The listing builds one solid part. Answer for the finished solid, in the listing's coordinates (mm). A direction names the side the tool comes from. Coordinates: 2 decimals unless noted, no trailing zeros. Order: outer loops, then holes, each group sorted by start corner. A loop starts at its lowest first (then second) coordinate and runs counter-clockwise, first axis right, second up. Notation, with made-up numbers: (29, 26.5) -> (63, 26.5) arc R22 cw to (63, 33.5) -> close; hole circle Ø3 at (74, 74.5). An arc over 180 degrees is marked (long way). One line per question, with ' | ' between items.
from build123d import *

# Parameters (mm, degrees)
F1_DEPTH = 5
F3_DEPTH = 185


with BuildPart() as f1:
    # F0 (on Front) → F1 (new body)
    with BuildSketch(Plane.XZ):
        with BuildLine():
            ThreePointArc((185, 30), (179.1421356237, 44.1421356237), (165, 50))
            Line((165, 50), (-165, 50))
            ThreePointArc((-165, 50), (-179.1421356237, 44.1421356237), (-185, 30))
            Line((-185, 30), (-185, -50))
            Line((-185, -50), (185, -50))
            Line((185, -50), (185, 30))
        make_face()
    extrude(amount=F1_DEPTH)

    # F2 (on Right) → F3 (join, symmetric)
    with BuildSketch(Plane.YZ):
        with BuildLine():
            ThreePointArc((12.3411369137, -50.3849132597), (12.1417214903, -49.9034818398), (11.6602900704, -49.7040664163))
            Line((11.6602900704, -49.7040664163), (-16.9780162429, -49.7040664163))
            ThreePointArc((-16.9780162429, -49.7040664163), (-17.4594476628, -49.9034818398), (-17.6588630863, -50.3849132597))
            Line((-17.6588630863, -50.3849132597), (-17.6588630863, -52.7040664163))
            Line((-17.6588630863, -52.7040664163), (12.3411369137, -52.7040664163))
            Line((12.3411369137, -52.7040664163), (12.3411369137, -50.3849132597))
        make_face()
    extrude(amount=F3_DEPTH, both=True)


solid = f1.part
Item 1: Section B-B, the plane z = 22.5 is taken. Give the vertices of the cut face in (x, y).
Computed values:
outline: (-185, -5) -> (185, -5) -> (185, 0) -> (-185, 0) -> close
Item 2: Section A-A, the plane x = 57 is taken. Give the vertices of the cut face in (y, z).
Computed values:
outline: (-17.66, -52.7) -> (12.34, -52.7) -> (12.34, -50.38) arc R0.68 ccw to (11.66, -49.7) -> (0, -49.7) -> (0, 50) -> (-5, 50) -> (-5, -49.7) -> (-16.98, -49.7) arc R0.68 ccw to (-17.66, -50.38) -> close
Item 3: Each of these flat-tipped pins is pushed along its axis until it touches: pin 1 Ø8 at (x, z) = (140.5, -2) entering from -Y; pin 2 Ø13 at (x, y) = (34.5, 7) entering from +Z; pin 3 Ø3 at (y, z) = (-7, -35) entering from +X. Where does it stop, or does it pass through?
Computed values:
pin 1: stops at y = -5 | pin 2: stops at z = -49.7 | pin 3: passes through
Item 4: For faces 1 (the face through (-178.986, -2.465, 44.297)), 2 (the face through (-3, 0, 1)), 3 (the face through (3, -11, -49.704)), determine the directions among +Z, -Z, +X, -X, +Y, -Y from which every point of the face is accessible in a straight line to the end or side of a thin tool.
Computed values:
face 1: +Z, -X, +Y, -Y | face 2: +Z, +X, -X, +Y | face 3: +Z, +X, -X, -Y
Item 5: Find the intervals of material crossed by L1, parallel to Y at x = -41.5, z = 14.5; L2, parallel to Z at x = -36, y = -7.5, in increasing order.
Computed values:
L1: y = -5 to 0 | L2: z = -52.7 to -49.7
Item 6: Section C-C, the plane y = 3.5 is taken. Give the vertices of the cut face in (x, z).
Computed values:
outline: (-185, -52.7) -> (185, -52.7) -> (185, -49.7) -> (-185, -49.7) -> close
